Design review of the part built by this model. Coordinates are the model's own, in mm. A direction names the side the tool comes from. Round coordinates to 2 decimals unless told otherwise and drop trailing zeros. Write each loop counter-clockwise with the first axis right and the second up, starting at its lowest first coordinate (ties: lowest second). Pieces come first, ordered by that corner, then holes. Notation, with made-up numbers: M -6.75,-35.75 L -2.75,-35.75 A8 cw -2.75,-26.75 Z; hole C -36,-19.5 d11. An arc over 180 degrees is marked long. Use CSV: the item, a comma, the result in double quotes.
from build123d import *

# Parameters (mm, degrees)
SKETCH1_W                    = 88.9
SKETCH1_H                    = 41.275
BOSS_EXTRUDE1_DEPTH          = 4.7625
SKETCH3_W                    = 12.7
SKETCH3_H                    = 41.275
BOSS_EXTRUDE2_DEPTH          = 4.7625
F_10_0_1935_DIAMETER_HOLE1_D = 4.9149
SKETCH9_W                    = 6.35
SKETCH9_H                    = 3.175
CUT_EXTRUDE1_DEPTH           = 50.924287989
FILLET1_R                    = 2.54
FILLET2_R                    = 2.54


with BuildPart() as part:
    # Sketch1 → Boss-Extrude1 (new body)
    with BuildSketch(Plane(origin=(0, 0, 0), x_dir=(1, 0, 0), z_dir=(0, 1, 0))):
        Rectangle(SKETCH1_W, SKETCH1_H)
    extrude(amount=BOSS_EXTRUDE1_DEPTH)

    # Sketch3 → Boss-Extrude2 (add)
    with BuildSketch(Plane.XZ):
        with Locations((38.1, 0)):
            Rectangle(SKETCH3_W, SKETCH3_H)
    extrude(amount=BOSS_EXTRUDE2_DEPTH)

    # #10 (0.1935) Diameter Hole1 (through all)
    with Locations(Plane(origin=(0, 4.7625, 0), x_dir=(1, 0, 0), z_dir=(0, 1, 0))):
        with Locations((38.1, 12.7), (38.1, -12.7)):
            Hole(F_10_0_1935_DIAMETER_HOLE1_D / 2)

    # Sketch9 → Cut-Extrude1 (cut, through all)
    with BuildSketch(Plane(origin=(0, 4.7625, 0), x_dir=(1, 0, 0), z_dir=(0, 1, 0))):
        with Locations((15.534707564, 19.05)):
            Rectangle(SKETCH9_W, SKETCH9_H)
        with Locations((-28.3765625, 19.05)):
            Rectangle(SKETCH9_W, SKETCH9_H)
        with Locations((-28.3765625, -19.05)):
            Rectangle(SKETCH9_W, SKETCH9_H)
        with Locations((15.534707564, -19.05)):
            Rectangle(SKETCH9_W, SKETCH9_H)
    extrude(amount=-CUT_EXTRUDE1_DEPTH, mode=Mode.SUBTRACT)

    # Fillet1
    fillet1_edges = [part.edges().sort_by_distance(p)[0] for p in [
        (31.75, 0, 0),
        (12.359707564, 2.38125, 20.6375),
        (18.709707564, 2.38125, 20.6375),
        (-31.5515625, 2.38125, 20.6375),
        (-25.2015625, 2.38125, 20.6375),
        (44.45, 0, 20.6375),
        (-44.45, 2.38125, 20.6375),
        (-31.5515625, 2.38125, -20.6375),
        (-25.2015625, 2.38125, -20.6375),
        (-44.45, 2.38125, -20.6375),
        (44.45, 0, -20.6375),
        (12.359707564, 2.38125, -20.6375),
        (18.709707564, 2.38125, -20.6375),
    ]]
    fillet(fillet1_edges, radius=FILLET1_R)

    # Fillet2
    fillet2_edges = [part.edges().sort_by_distance(p)[0] for p in [
        (18.709707564, 2.38125, -17.4625),
        (12.359707564, 2.38125, -17.4625),
        (-31.5515625, 2.38125, -17.4625),
        (-25.2015625, 2.38125, -17.4625),
        (-25.2015625, 2.38125, 17.4625),
        (-31.5515625, 2.38125, 17.4625),
        (12.359707564, 2.38125, 17.4625),
        (18.709707564, 2.38125, 17.4625),
    ]]
    fillet(fillet2_edges, radius=FILLET2_R)


solid = part.part
1) Add section A-A on z = 12.7. Write out the cut boundary in (x, y).
Answers:
outline,"M -44.45,0 L 29.21,0 A2.54 cw 31.75,-2.54 L 31.75,-4.76 L 35.64,-4.76 L 35.64,4.76 L -44.45,4.76 Z; M 40.56,-4.76 L 44.45,-4.76 L 44.45,4.76 L 40.56,4.76 Z"
2) Machinability: for faces 4 (the face through (-24.06, 2.35, 20.22)), 5 (the face through (-24.1, 2.35, -20.19)), 6 (the face through (39.91, -0.07, -14.36)), which of the approach directions +Z, -Z, +X, -X, +Y, -Y give a long, thin tool a straight path to every point of the face, cutting with its end or side? Answer none if there is none.
Answers:
face 4,"+Z, +Y, -Y"
face 5,"-Z, +Y, -Y"
face 6,"+Y, -Y"
3) The part is to be moulded in two halves that separate along X. For faces 1 (the face through (43.7, -0.1, -19.9)), 2 (the face through (-32.65, 2.35, 20.19)), 3 (the face through (34, 1, 20.638)), say which applies: released by +X, released by -X, zero draft, split by the parting line, or undercut.
Answers:
face 1,"released by +X"
face 2,"undercut"
face 3,"zero draft"
4) Add section C-C on z = 8. Write out the cut boundary in (x, y).
Answers:
outline,"M -44.45,0 L 29.21,0 A2.54 cw 31.75,-2.54 L 31.75,-4.76 L 44.45,-4.76 L 44.45,4.76 L -44.45,4.76 Z"
5) Wall thickness on line 1 along Z through (x, y) = (38.1, 1.5); line 2 along X through (y, z) = (2.5, -12.7); line 3 along Y through (x, z) = (24, -8): over which ranges is each line inside the solid? List them lowest first. Write a range as [from, to].
Answers:
line 1,"[-20.64, -15.16], [-10.24, 10.24], [15.16, 20.64]"
line 2,"[-44.45, 35.64], [40.56, 44.45]"
line 3,"[0, 4.76]"
6) For pin 1 Ø1.6 at (x, y) = (-28, 2) entering from -Z; pin 2 Ø1.5 at (x, z) = (11.5, -7.5) entering from -Y; pin 3 Ø0.7 at (y, z) = (-3, -1) entering from -X; pin 4 Ø4.5 at (x, z) = (38.1, 12.7) entering from +Y, all flat-tipped, find the tip position at first contact; note any pin that passes through.
Answers:
pin 1,"z = -17.47"
pin 2,"y = 0"
pin 3,"x = 31.75"
pin 4,"through"
7) Add section B-B on x = 38.1. Write out the cut boundary in (y, z).
Answers:
outline,"M -4.76,-20.64 L 4.76,-20.64 L 4.76,-15.16 L -4.76,-15.16 Z; M -4.76,-10.24 L 4.76,-10.24 L 4.76,10.24 L -4.76,10.24 Z; M -4.76,15.16 L 4.76,15.16 L 4.76,20.64 L -4.76,20.64 Z"
8) Add section D-D on y = 1.5. Give the number of separate pieces and of enclosed holes in the cut face, then the cut area to 3 significant figures.
Answers:
separate pieces,"1"
enclosed holes,"2"
area,"3,540 mm²"
